Can you work these out from the model? Positions are in its coordinate system, mm. Give positions to 0.01 mm unless a question says otherwise; leave off trailing zeros. Order: outer loops, then holes, each group sorted by start corner. A loop starts at its lowest first (then second) coordinate and runs counter-clockwise, first axis right, second up. Notation, with made-up numbers: (87.25, -12.75) - (93.25, -12.75) arc R23 ccw to (93.25, 12.25) - close; hole circle Ø6 at (8.5, 9). An arc over 180 degrees is marked (long way). Return JSON: item names as keys, results as strings.
```python
from build123d import *

# Parameters (mm, degrees)
SKETCH_1_W          = 50
SKETCH_1_H          = 50
EXTRUDE_1_DEPTH     = 2
SKETCH_3_W          = 76.549088161
SKETCH_3_H          = 63.496312915
CUT_EXTRUDE_3_DEPTH = 10
M3X0_5_1_D          = 2.5
M3X0_5_1_DEPTH      = 8.5
M3X0_5_1_TIP        = 0.751075774


with BuildPart() as part:
    # ｽｹｯﾁ1 → ﾎﾞｽ - 押し出し1 (new body)
    with BuildSketch(Plane.XY):
        Rectangle(SKETCH_1_W, SKETCH_1_H)
    extrude(amount=EXTRUDE_1_DEPTH)

    # ｽｹｯﾁ3 → ｶｯﾄ - 押し出し3 (cut)
    with BuildSketch(Plane.XY.offset(2)):
        with Locations((-0.951764861, 3.501134841)):
            Rectangle(SKETCH_3_W, SKETCH_3_H)
        Polygon((14.5, -4.5), (4.5, -25), (-4.5, -25), (-4.5, 4.5), (14.5, 4.5), align=None, mode=Mode.SUBTRACT)
    extrude(amount=-CUT_EXTRUDE_3_DEPTH, mode=Mode.SUBTRACT)

    # M3x0.5 ねじ穴1
    with Locations(Plane.XY.offset(2)):
        with Locations((0, 0), (10, 0), (0, -9.51), (0, -19.51)):
            Hole(M3X0_5_1_D / 2, depth=M3X0_5_1_DEPTH)
            with Locations((0, 0, -(M3X0_5_1_DEPTH + M3X0_5_1_TIP / 2))):  # 118° drill point
                Cone(0, M3X0_5_1_D / 2, M3X0_5_1_TIP, mode=Mode.SUBTRACT)


solid = part.part
```
1. Suppose I cut it at B-B (y = 0). List the corners of the cut face in (x, z) for me.
Checks:
{"outline": "(-4.5, 0) - (-1.25, 0) - (-1.25, 2) - (-4.5, 2) - close; (1.25, 0) - (8.75, 0) - (8.75, 2) - (1.25, 2) - close; (11.25, 0) - (14.5, 0) - (14.5, 2) - (11.25, 2) - close"}
2. Suppose I cut it at A-A (z = 1.45). List the corners of the cut face in (x, y) for me.
Checks:
{"outline": "(-4.5, -25) - (4.5, -25) - (14.5, -4.5) - (14.5, 4.5) - (-4.5, 4.5) - close; hole circle Ø2.5 at (0, -19.51); hole circle Ø2.5 at (0, -9.51); hole circle Ø2.5 at (0, 0); hole circle Ø2.5 at (10, 0)"}
3. Suppose I cut it at D-D (y = -19.51). List the corners of the cut face in (x, z) for me.
Checks:
{"outline": "(-4.5, 0) - (-1.25, 0) - (-1.25, 2) - (-4.5, 2) - close; (1.25, 0) - (7.18, 0) - (7.18, 2) - (1.25, 2) - close"}
4. Suppose I cut it at C-C (x = 0). List the corners of the cut face in (y, z) for me.
Checks:
{"outline": "(-25, 0) - (-20.76, 0) - (-20.76, 2) - (-25, 2) - close; (-18.26, 0) - (-10.76, 0) - (-10.76, 2) - (-18.26, 2) - close; (-8.26, 0) - (-1.25, 0) - (-1.25, 2) - (-8.26, 2) - close; (1.25, 0) - (4.5, 0) - (4.5, 2) - (1.25, 2) - close"}
5. Thinking about a two-plate mould opening in Y: for faces 1 (the face through (3, -10, 2)), 2 (the face through (0.27, -20.73, 0.99)), 3 (the face through (5, 4.5, 1)), which applies, +Y half, -Y half, draft (parallel to the pull), parting line (faces both ways), or undercut?
Checks:
{"face 1": "draft", "face 2": "undercut", "face 3": "+Y half"}
6. If I drill on L1, parallel to Y at x = 0, z = 1.25; L2, parallel to Y at x = 10, z = 1 (3 decimals); L3, parallel to X at y = -19.5, z = 0.35, over which ranges is the centre line in solid material (lowest first)? Write a range as [from, to].
Checks:
{"L1": "[-25, -20.76], [-18.26, -10.76], [-8.26, -1.25], [1.25, 4.5]", "L2": "[-13.725, -1.25], [1.25, 4.5]", "L3": "[-4.5, -1.25], [1.25, 7.18]"}
7. For pin 1 Ø2 at (x, y) = (0, -19.51) entering from +Z, with a flat end and sliding along its axis, tell me the tip position at first contact or that it passes through.
Checks:
{"pin 1": "through"}
